Design review of the part built by this model. Coordinates are the model's own, in mm. A direction names the side the tool comes from. Coordinates: 2 decimals unless noted, no trailing zeros. Loops run counter-clockwise (first coordinate to the right, second up) from the corner with the lowest first, then second, coordinate; pieces in that order, holes last. Notation, with made-up numbers: (60, 57) - (86, 57) arc R21 ccw to (86, 71) - close; hole circle Ø1 at (-7.5, 11). An arc over 180 degrees is marked (long way). One line per question, with ' | ' between items.
from build123d import *

# Parameters (mm, degrees)
EXTRUDE_1_DEPTH = 1.5
SKETCH_2_W      = 4.318
SKETCH_2_H      = 5.334
EXTRUDE_2_DEPTH = 1.5
SKETCH_3_W      = 6.223
SKETCH_3_H      = 5.08
EXTRUDE_3_DEPTH = 8.75
FILLET_1_R      = 1
FILLET_2_R      = 2


with BuildPart() as part:
    # 草图1 → 凸台-拉伸1 (new body)
    with BuildSketch(Plane.XY):
        with BuildLine():
            Line((90.932, 85.09), (91.186, 85.344))
            Line((91.186, 85.344), (91.186, 90.424))
            Line((91.186, 90.424), (97.162789, 90.424))
            ThreePointArc((97.162789, 90.424), (97.51649159, 90.57050841), (97.663, 90.924211))
            Line((97.663, 90.924211), (97.663, 94.361))
            Line((97.663, 94.361), (106.934, 94.361))
            Line((106.934, 94.361), (107.696, 93.599))
            Line((107.696, 93.599), (107.696, 83.312))
            Line((107.696, 83.312), (107.442, 83.058))
            Line((107.442, 83.058), (102.616, 83.058))
            Line((102.616, 83.058), (102.616, 76.833545254))
            Line((102.616, 76.833545254), (95.758, 76.833545254))
            Line((95.758, 76.833545254), (95.758, 75.946))
            Line((95.758, 75.946), (90.932, 75.946))
            Line((90.932, 75.946), (90.932, 85.09))
        make_face()
    extrude(amount=EXTRUDE_1_DEPTH)

    # 草图2 → 凸台-拉伸2 (add)
    with BuildSketch(Plane.XY):
        with Locations((93.091, 78.613)):
            Rectangle(SKETCH_2_W, SKETCH_2_H)
    extrude(amount=-EXTRUDE_2_DEPTH)

    # 草图3 → 凸台-拉伸3 (add)
    with BuildSketch(Plane.XY):
        with Locations((94.2975, 87.884)):
            Rectangle(SKETCH_3_W, SKETCH_3_H)
    extrude(amount=-EXTRUDE_3_DEPTH)

    # 圆角1
    # the kernel refuses this fillet: 1 mm, written as the material it adds along each edge
    with BuildSketch(Plane(origin=(91.186, 85.344, 0), x_dir=(-0.7071067811889411, -0.7071067811841542, 0), z_dir=(0, 0, 1))) as fillet_1_piece_1:
        with BuildLine():
            CenterArc((0.415817011, -0.998396551), FILLET_1_R, 93.245063402, 41.754936598)
            Line((-0.29128977, -0.29128977), (0, 0))
            Line((0, 0), (0.359210245, 0))
        make_face()
    extrude(amount=1.5)

    # 圆角2
    # the kernel refuses this fillet: 2 mm, written as the material it adds along each edge
    with BuildSketch(Plane(origin=(95.758, 76.833545254, 0), x_dir=(1, 0, 0), z_dir=(0, 0, 1))) as fillet_2_piece_1:
        with BuildLine():
            CenterArc((1.662060299, -2), FILLET_2_R, 90, 56.204705158)
            Line((0, -0.887545254), (-0.033241206, -0.86529616))
            ThreePointArc((-0.033241206, -0.86529616), (-0.04, -0.443772627), (-0.04, 0))
            Line((-0.04, 0), (0, 0.04))
            Line((0, 0.04), (1.662060299, 0.04))
            Line((1.662060299, 0.04), (1.662060299, 0))
        make_face()
    extrude(amount=1.5)


solid = part.part
Q1. To check wall thickness, follow line 1 along Y through (x, z) = (96.25, -6); line 2 along Z through (x, y) = (98.5, 90.5); line 3 along Y through (x, z) = (101, 0.75). State the ranges of each line that lie inside material, in increasing order.
Returned:
line 1: y = 85.34 to 90.42 | line 2: z = 0 to 1.5 | line 3: y = 76.83 to 94.36
Q2. Take a section at B-B (y = 87.5). Give the boundary of the cut face in (x, z).
Returned:
outline: (91.19, -8.75) - (97.41, -8.75) - (97.41, 0) - (107.7, 0) - (107.7, 1.5) - (91.19, 1.5) - close
Q3. For pin 1 (0.8 mm diameter, centred on x = 105, z = 1, fed in from -Y); pin 2 (1.5 mm diameter, centred on x = 93.5, z = -0.5, fed in from +Y); pin 3 (4.5 mm diameter, centred on x = 93, y = 79, fed in from -Z), all flat-tipped, find the tip position at first contact; note any pin that passes through.
Returned:
pin 1: stops at y = 83.06 | pin 2: stops at y = 90.42 | pin 3: stops at z = -1.5
Q4. Tool access review of faces 5 (the flat face through (93, 79, -1.5)), 6 (the flat face through (100, 76.834, 1)), 7 (the flat face through (97.663, 93, 1)), 8 (the flat face through (94, 85.344, -4)), 9 (the flat face through (95.25, 79, -1)): name each direction out of +Z, -Z, +X, -X, +Y, -Y from which nothing blocks a thin tool from reaching the whole face with its end or side.
Returned:
face 5: -Z, +X, -X, -Y | face 6: +Z, -Z, +X, -Y | face 7: +Z, -Z, -X, +Y | face 8: -Z, +X, -X | face 9: -Z, +X, -Y
Q5. Draft analysis for pull direction Y (two halves, no side actions). For faces 1 (the flat face through (93, 81.28, -1)), 2 (the flat face through (105, 83.058, 1)), 3 (the flat face through (97.409, 88, -4)), 4 (the flat face through (94, 90.424, -4)), state which applies: +Y half, -Y half, draft (parallel to the pull), parting line (faces both ways), or undercut.
Returned:
face 1: undercut | face 2: -Y half | face 3: draft | face 4: +Y half
Q6. Take a section at A-A (x = 93.75). Give the boundary of the cut face in (y, z).
Returned:
outline: (75.95, -1.5) - (81.28, -1.5) - (81.28, 0) - (85.34, 0) - (85.34, -8.75) - (90.42, -8.75) - (90.42, 1.5) - (75.95, 1.5) - close
Q7. Take a section at C-C (z = 0.5). Give the boundary of the cut face in (x, y).
Returned:
outline: (90.93, 75.95) - (95.76, 75.95) arc R2 cw to (97.42, 76.83) - (102.62, 76.83) - (102.62, 83.06) - (107.44, 83.06) - (107.7, 83.31) - (107.7, 93.6) - (106.93, 94.36) - (97.66, 94.36) - (97.66, 90.92) arc R0.5 cw to (97.16, 90.42) - (91.19, 90.42) - (91.19, 85.76) arc R1 cw to (90.93, 85.09) - close
Q8. Take a section at D-D (y = 79.75). Give the boundary of the cut face in (x, z).
Returned:
outline: (90.93, -1.5) - (95.25, -1.5) - (95.25, 0) - (102.62, 0) - (102.62, 1.5) - (90.93, 1.5) - close
